Read the model definition and answer for the solid it produces. Units are mm, in the model's axes. Give positions to 0.01 mm unless a question says otherwise; leave off trailing zeros. Loops run counter-clockwise (first coordinate to the right, second up) from the corner with the lowest first, then second, coordinate; pieces in that order, holes last. Notation, with made-up numbers: (-34.75, 47.25) - (-8.75, 47.25) arc R23 ccw to (-8.75, 78.25) - close; hole circle Ø2 at (87.25, 89). An arc over 180 degrees is marked (long way). Use a Markdown table: item, result. Add a question column.
Item 1: Consider probe 1 along Y at (x, z) = (0, 27); probe 2 along Y at (x, z) = (-11, 43); probe 3 along X at (y, z) = (-16, 45.5) (3 decimals). Determine where each line is inside the solid, lowest interval first. Write a range as [from, to].
Item 2: Each of these flat-tipped pins is pushed along its axis until it touches: P1, Ø1.5, axis at x = -6, z = 8.5, coming from the +Y side; P2, Ø3, axis at x = 2, z = 17, coming from the -Y side (3 decimals); P3, Ø6, axis at y = -4.5, z = 23.5, coming from the +X side (3 decimals). Where does it stop, or does it pass through?
Item 3: A cutting plane is placed at C-C (z = 23.5). Determine the outline of the cut face in (x, y) (3 decimals).
Item 4: A cutting plane is placed at A-A (y = 8). Determine the outline of the cut face in (x, z).
Item 5: For a pull along X with two mould halves and no side action, classify faces 1 (the face through (16.22, -0.23, 24.65)), 2 (the face through (14.28, -0.23, 25.35)), 3 (the face through (-16.22, -0.23, 24.65)) as +X half, -X half, draft (parallel to the pull), parting line (faces both ways), or undercut.
from build123d import *

# Parameters (mm, degrees)
PAD_DEPTH          = 18.5
PAD_DEPTH_BACK     = 18.5
POLARPATTERN_COUNT = 4
POCKET_DEPTH       = 6.4748338525
POCKET001_DEPTH    = 6.4748338525
POCKET002_DEPTH    = 1.9919488777
POCKET003_DEPTH    = 5
POCKET004_DEPTH    = 5
POCKET005_DEPTH    = 5
POCKET006_DEPTH    = 5
POCKET007_DEPTH    = 5
POCKET008_DEPTH    = 5


with BuildPart() as part:
    # Sketch → Pad (new body, two sides)
    with BuildSketch(Plane.XZ) as pad_sk:
        Polygon((-16.5, 50), (-12, 0), (-14, 0), (-18.5, 50), align=None)
    pad = extrude(amount=PAD_DEPTH) + extrude(pad_sk.sketch, amount=-PAD_DEPTH_BACK)

    # PolarPattern: Pad ×4 about axis
    polarpattern_axis = Axis((0, 0, 0), (0, 0, 1))
    for i in range(1, POLARPATTERN_COUNT):
        add(pad.rotate(polarpattern_axis, i * 360 / POLARPATTERN_COUNT))

    # PolarPattern Face15 → Pocket (cut, through all)
    with BuildSketch(Plane(origin=(-13.5, -17, 16.6666666667), x_dir=(0, -1, 0), z_dir=(0.9959744388, 0, 0.0896376995))):
        Polygon((-3, 16.73403053), (1.5, -33.4680610599), (1.5, 16.73403053), align=None)
    extrude(amount=-POCKET_DEPTH, mode=Mode.SUBTRACT)

    # Pocket Face11 → Pocket001 (cut, through all)
    with BuildSketch(Plane(origin=(-17, -13.5, 16.6666666667), x_dir=(1, 0, 0), z_dir=(0, 0.9959744388, 0.0896376995))):
        Polygon((-1.5, 16.73403053), (-1.5, -33.4680610599), (3, 16.73403053), align=None)
    extrude(amount=-POCKET001_DEPTH, mode=Mode.SUBTRACT)

    # Pocket001 Face4 → Pocket002 (cut)
    with BuildSketch(Plane(origin=(-15.5, 17, 16.6666666667), x_dir=(0, 1, 0), z_dir=(-0.9959744388, 0, -0.0896376995))):
        Polygon((1.5, -33.4680610599), (1.5, 16.73403053), (-3, 16.73403053), align=None)
    extrude(amount=-POCKET002_DEPTH, mode=Mode.SUBTRACT)

    # Pocket002 Face9 → Pocket003 (cut)
    with BuildSketch(Plane(origin=(-17, 13.5, 16.6666666667), x_dir=(-1, 0, 0), z_dir=(0, -0.9959744388, 0.0896376995))):
        Polygon((-3, 16.73403053), (1.5, -33.4680610599), (1.5, 16.73403053), align=None)
    extrude(amount=-POCKET003_DEPTH, mode=Mode.SUBTRACT)

    # Pocket003 Face15 → Pocket004 (cut)
    with BuildSketch(Plane(origin=(13.5, -17, 16.6666666667), x_dir=(0, 1, 0), z_dir=(-0.9959744388, 0, 0.0896376995))):
        Polygon((-1.5, 16.73403053), (-1.5, -33.4680610599), (3, 16.73403053), align=None)
    extrude(amount=-POCKET004_DEPTH, mode=Mode.SUBTRACT)

    # Pocket004 Face26 → Pocket005 (cut)
    with BuildSketch(Plane(origin=(13.5, 17, 16.6666666667), x_dir=(0, 1, 0), z_dir=(-0.9959744388, 0, 0.0896376995))):
        Polygon((-3, 16.73403053), (1.5, -33.4680610599), (1.5, 16.73403053), align=None)
    extrude(amount=-POCKET005_DEPTH, mode=Mode.SUBTRACT)

    # Pocket005 Face21 → Pocket006 (cut)
    with BuildSketch(Plane(origin=(17, 13.5, 16.6666666667), x_dir=(-1, 0, 0), z_dir=(0, -0.9959744388, 0.0896376995))):
        Polygon((-1.5, 16.73403053), (-1.5, -33.4680610599), (3, 16.73403053), align=None)
    extrude(amount=-POCKET006_DEPTH, mode=Mode.SUBTRACT)

    # Pocket006 Face19 → Pocket007 (cut)
    with BuildSketch(Plane(origin=(17, -13.5, 16.6666666667), x_dir=(1, 0, 0), z_dir=(0, 0.9959744388, 0.0896376995))):
        Polygon((-3, 16.73403053), (1.5, -33.4680610599), (1.5, 16.73403053), align=None)
    extrude(amount=-POCKET007_DEPTH, mode=Mode.SUBTRACT)

    # Pocket007 Face2 → Pocket008 (cut)
    with BuildSketch(Plane(origin=(-13.0080349172, 16.25, 0.0892768575), x_dir=(0, 1, 0), z_dir=(-0.0896376995, 0, 0.9959744388))):
        Polygon((2.25, 0.9959744388), (-2.25, 0.9959744388), (-2.25, -0.9959744388), (-2.2339301657, -0.9959744388), (2.25, -0.9959744388), align=None)
    extrude(amount=-POCKET008_DEPTH, mode=Mode.SUBTRACT)


solid = part.part
Geometry says:
| question | item | result |
|---|---|---|
| 1 | probe 1 | [-16.43, -14.43], [14.43, 16.43] |
| 1 | probe 2 | [-17.87, -15.87], [15.87, 17.87] |
| 1 | probe 3 | [-18.095, -16.095], [16.095, 18.095] |
| 2 | P1 | y = 14.83 |
| 2 | P2 | y = -15.665 |
| 2 | P3 | x = 16.385 |
| 3 | outline | (-16.131, -16.115) - (-16.115, -16.115) - (-16.115, -16.131) - (-14.115, -16.115) - (14.115, -16.115) - (16.115, -16.131) - (16.115, -16.115) - (16.131, -16.115) - (16.115, -14.115) - (16.115, 14.115) - (16.131, 16.115) - (16.115, 16.115) - (16.115, 16.131) - (14.115, 16.115) - (-14.115, 16.115) - (-14.115, 16.099) - (-16.115, 16.115) - (-16.131, 16.115) - (-16.115, 14.115) - (-16.115, -14.115) - close; hole (-14.115, -14.115) - (14.115, -14.115) - (14.115, 14.115) - (-14.115, 14.115) - close |
| 4 | outline | (-18.5, 50) - (-14, 0) - (-12, 0) - (-16.5, 50) - close; (12, 0) - (14, 0) - (18.5, 50) - (16.5, 50) - close |
| 5 | face 1 | +X half |
| 5 | face 2 | undercut |
| 5 | face 3 | -X half |
